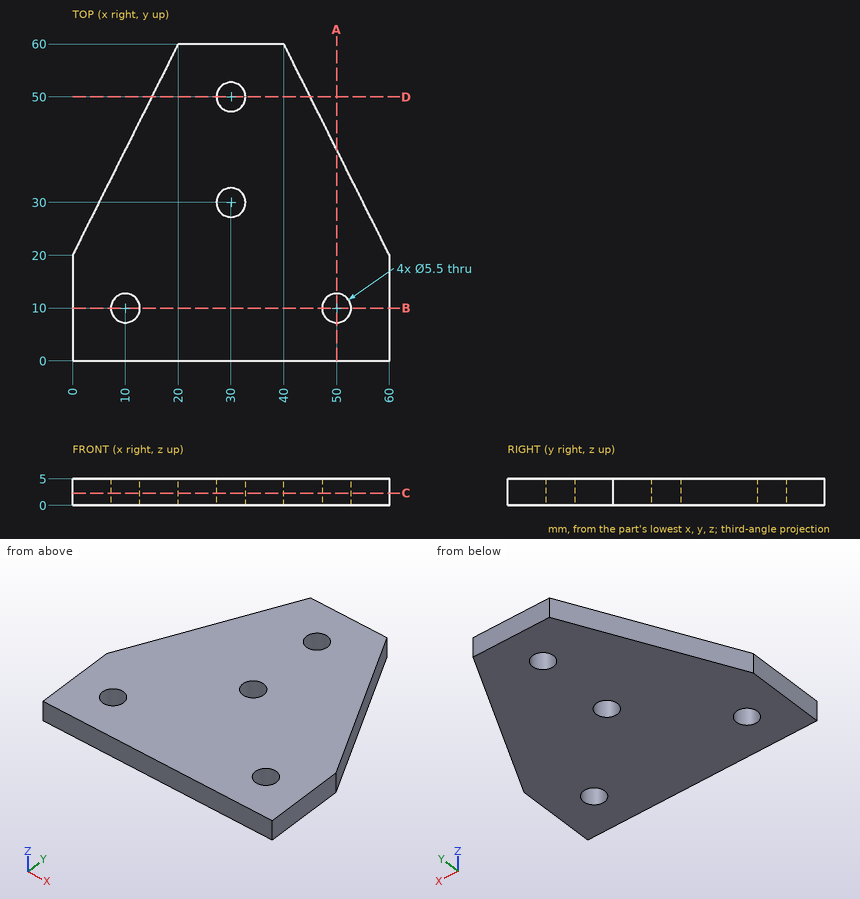
Here's the drawing with two shaded views (mm, measured from the low corner). I have some questions. Round coordinates to 2 decimals unless told otherwise and drop trailing zeros. Loops run counter-clockwise (first coordinate to the right, second up) from the corner with the lowest first, then second, coordinate; pieces in that order, holes last. Notation, with made-up numbers: (-37.5, 27) - (-6.5, 27) arc R34 ccw to (-6.5, 57) - close; hole circle Ø4 at (9.25, 64). An arc over 180 degrees is marked (long way). Use CSV: the item, a comma, the result in double quotes. Start each with the question number.
1) Please list where these lines run through material, in increasing order: probe 1 along Y at (x, z) = (30, 1.05); probe 2 along Y at (x, z) = (50, 1.45); probe 3 along X at (y, z) = (9, 2.7). Write a range as [from, to].
2) If we section it at B-B on y = 10: Write out the boundary of the cut face in (x, z), plus the area to 3 significant figures.
3) If we section it at D-D on y = 50: Write out the boundary of the cut face in (x, z).
4) If we section it at A-A on x = 50: Write out the boundary of the cut face in (y, z), plus the area to 4 significant figures.
5) If we section it at C-C on z = 2.35: Write out the boundary of the cut face in (x, y), plus the area to 3 significant figures.
Geometry results:
1,probe 1,"y = [0, 27.25], [32.75, 47.25], [52.75, 60]"
1,probe 2,"y = [0, 7.25], [12.75, 40]"
1,probe 3,"x = [0, 7.44], [12.56, 47.44], [52.56, 60]"
2,outline,"(0, 0) - (7.25, 0) - (7.25, 5) - (0, 5) - close; (12.75, 0) - (47.25, 0) - (47.25, 5) - (12.75, 5) - close; (52.75, 0) - (60, 0) - (60, 5) - (52.75, 5) - close"
2,area,"245 mm2"
3,outline,"(15, 0) - (27.25, 0) - (27.25, 5) - (15, 5) - close; (32.75, 0) - (45, 0) - (45, 5) - (32.75, 5) - close"
4,outline,"(0, 0) - (7.25, 0) - (7.25, 5) - (0, 5) - close; (12.75, 0) - (40, 0) - (40, 5) - (12.75, 5) - close"
4,area,"172.5 mm2"
5,outline,"(0, 0) - (60, 0) - (60, 20) - (40, 60) - (20, 60) - (0, 20) - close; hole circle Ø5.5 at (10, 10); hole circle Ø5.5 at (30, 30); hole circle Ø5.5 at (30, 50); hole circle Ø5.5 at (50, 10)"
5,area,"2,700 mm2"
